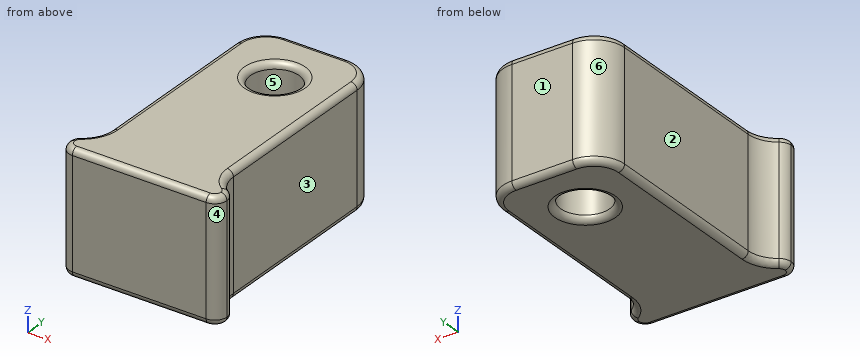
```python
from build123d import *

# Parameters (mm, degrees)
F0_R     = 4
F1_DEPTH = 20
F2_R     = 5
F3_R     = 1.99999
F4_R     = 5
F5_R     = 1


# Not quite as in the source:
# - a fillet or chamfer is up to 0.001 mm smaller than in the source, because OpenCascade refuses the exact size


with BuildPart() as f1:
    # F0 (on Top) → F1 (new body)
    with BuildSketch(Plane.XY):
        Polygon((-10, -20.75), (10, -20.75), (13, -20.75), (13, -16.75), (10, -16.75), (10, 20.75), (-10, 20.75), (-10, -16.75), (-13, -16.75), (-13, -20.75), align=None)
        with Locations((0, 10.75)):
            Circle(F0_R, mode=Mode.SUBTRACT)
    extrude(amount=F1_DEPTH)

    # F2
    f2_edges = [f1.edges().sort_by_distance(p)[0] for p in [
        (-10, 20.75, 10),
        (10, 20.75, 10),
    ]]
    fillet(f2_edges, radius=F2_R)

    # F3 (radius 2 in the source; OpenCascade refuses exactly that, so slightly less here)
    f3_edges = [f1.edges().sort_by_distance(p)[0] for p in [
        (-13, -16.75, 10),
        (-13, -20.75, 10),
        (13, -16.75, 10),
        (13, -20.75, 10),
    ]]
    fillet(f3_edges, radius=F3_R)

    # F4
    f4_edges = [f1.edges().sort_by_distance(p)[0] for p in [
        (-10, -16.75, 10),
        (10, -16.75, 10),
    ]]
    fillet(f4_edges, radius=F4_R)

    # F5
    f5_edges = [f1.edges().sort_by_distance(p)[0] for p in [
        (12.772811, -17.824174, 20),
        (10.567975, -15.319984, 20),
        (13, -18.75, 20),
        (10, 1.372284, 20),
        (12.414216, -20.164216, 20),
        (8.535534, 19.285534, 20),
        (0, -20.75, 20),
        (0, 20.75, 20),
        (-12.414216, -20.164216, 20),
        (-8.535534, 19.285534, 20),
        (-13, -18.75, 20),
        (-10, 1.372284, 20),
        (-12.772811, -17.824174, 20),
        (-10.567975, -15.319984, 20),
        (-4, 10.75, 20),
        (12.772811, -17.824174, 0),
        (10.567975, -15.319984, 0),
        (13, -18.75, 0),
        (10, 1.372284, 0),
        (12.414216, -20.164216, 0),
        (8.535534, 19.285534, 0),
        (0, -20.75, 0),
        (0, 20.75, 0),
        (-12.414216, -20.164216, 0),
        (-8.535534, 19.285534, 0),
        (-13, -18.75, 0),
        (-10, 1.372284, 0),
        (-12.772811, -17.824174, 0),
        (-10.567975, -15.319984, 0),
        (-4, 10.75, 0),
    ]]
    fillet(f5_edges, radius=F5_R)


solid = f1.part
```
Can you work these out from the model? Positions are in its coordinate system, mm. Face numbers are marked on the shaded views. A direction names the side the tool comes from. Round coordinates to 2 decimals unless told otherwise and drop trailing zeros. Loops run counter-clockwise (first coordinate to the right, second up) from the corner with the lowest first, then second, coordinate; pieces in that order, holes last. Notation, with made-up numbers: M 65.25,52 L 103.25,52 A11 ccw 103.25,59 Z; hole C 74.25,54.5 d9. An arc over 180 degrees is marked long. Write item = value, one per line. Start each with the question number.
(1) Suppose I cut it at C-C on y = -8.5. Write out the boundary of the cut face in (x, z).
(2) Which directions (+Z, -Z, +X, -X, +Y, -Y) give clear straight access to the entire face, cutting with the end or side of a thin tool? Please do the marked faces 1, 2 and 3.
(3) Suppose I cut it at A-A on x = 0. Write out the boundary of the cut face in (y, z).
(4) I'm going to push flat-ended pins straight in: P1, Ø1.5, axis at y = -14.5, z = 4.5, coming from the +X side; P2, Ø6, axis at y = -11.5, z = 8.5, coming from the +X side; P3, Ø12, axis at y = 3.5, z = 14.5, coming from the +X side. Where does each tip first touch, or does it pass through?
(5) Suppose I cut it at B-B on y = 10.75. Write out the boundary of the cut face in (x, z).
(6) If we mould it in two halves opening along X, with no side actions, what happens to the marked faces 4, 5 and 6? For each: released by +X, released by -X, zero draft, split by the parting line, or undercut.
(7) I need wall thicknesses on line 1 along X through (y, z) = (11, 7.75); line 2 along Y through (x, z) = (0, 14.75); line 3 along Y through (x, z) = (8, 8). Which ranges of each line are inside material? Lowest first, please.
Answer block:
q1.outline = M -10,1 A1 ccw -9,0 L 9,0 A1 ccw 10,1 L 10,19 A1 ccw 9,20 L -9,20 A1 ccw -10,19 Z
q2.face_1 = +Z, -Z, +X, -X, +Y
q2.face_2 = +Z, -Z, -X, +Y
q2.face_3 = +Z, -Z, +X, +Y
q3.outline = M -20.75,1 A1 ccw -19.75,0 L 5.75,0 A1 ccw 6.75,1 L 6.75,19 A1 ccw 5.75,20 L -19.75,20 A1 ccw -20.75,19 Z; M 14.75,1 A1 ccw 15.75,0 L 19.75,0 A1 ccw 20.75,1 L 20.75,19 A1 ccw 19.75,20 L 15.75,20 A1 ccw 14.75,19 Z
q4.P1 = 10.53
q4.P2 = 10.23
q4.P3 = 10
q5.outline = M -10,1 A1 ccw -9,0 L -5,0 A1 ccw -4,1 L -4,19 A1 ccw -5,20 L -9,20 A1 ccw -10,19 Z; M 4,1 A1 ccw 5,0 L 9,0 A1 ccw 10,1 L 10,19 A1 ccw 9,20 L 5,20 A1 ccw 4,19 Z
q6.face_4 = released by +X
q6.face_5 = undercut
q6.face_6 = released by -X
q7.line_1 = -10 to -3.99, 3.99 to 10
q7.line_2 = -20.75 to 6.75, 14.75 to 20.75
q7.line_3 = -20.75 to 19.75
